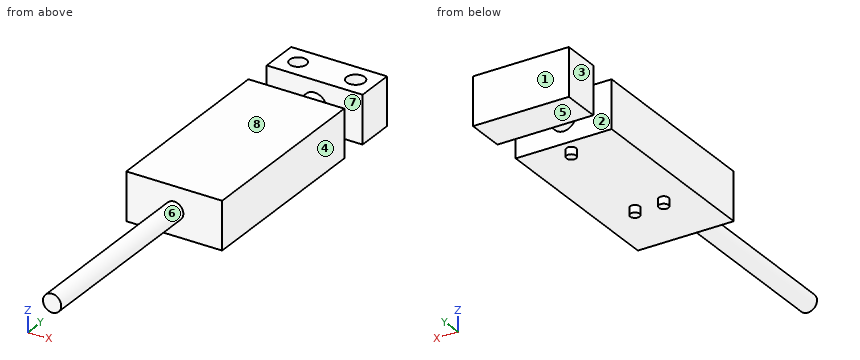
```python
from build123d import *

# Parameters (mm, degrees)
SKETCH1_W           = 200
SKETCH1_H           = 400
BOSS_EXTRUDE1_DEPTH = 100
SKETCH2_R           = 25
BOSS_EXTRUDE2_DEPTH = 60
SKETCH3_W           = 200
SKETCH3_H           = 100
BOSS_EXTRUDE3_DEPTH = 80
SKETCH4_R           = 17.5
SKETCH4_R_2         = 18.82666719
CUT_EXTRUDE1_DEPTH  = 40
SKETCH5_R           = 19
BOSS_EXTRUDE4_DEPTH = 400
SKETCH7_R           = 10
BOSS_EXTRUDE5_DEPTH = 15


with BuildPart() as part:
    # Sketch1 → Boss-Extrude1 (new body)
    with BuildSketch(Plane.XY):
        Rectangle(SKETCH1_W, SKETCH1_H)
    extrude(amount=BOSS_EXTRUDE1_DEPTH)

    # Sketch2 → Boss-Extrude2 (add)
    with BuildSketch(Plane(origin=(0, 200, 0), x_dir=(1, 0, 0), z_dir=(0, 1, 0))):
        with Locations(Location((0, -50, 0), (0, 0, 90))):
            Circle(SKETCH2_R)
    extrude(amount=BOSS_EXTRUDE2_DEPTH)

    # Sketch3 → Boss-Extrude3 (add)
    with BuildSketch(Plane(origin=(0, 260, 0), x_dir=(1, 0, 0), z_dir=(0, 1, 0))):
        with Locations((0, -50)):
            Rectangle(SKETCH3_W, SKETCH3_H)
    extrude(amount=BOSS_EXTRUDE3_DEPTH)

    # Sketch4 → Cut-Extrude1 (cut)
    with BuildSketch(Plane.XY.offset(100)):
        with Locations((-60, 300)):
            Circle(SKETCH4_R)
        with Locations((60, 300)):
            Circle(SKETCH4_R_2)
    extrude(amount=-CUT_EXTRUDE1_DEPTH, mode=Mode.SUBTRACT)

    # Sketch5 → Boss-Extrude4 (add)
    with BuildSketch(Plane.XZ.offset(200)):
        with Locations(Location((0, 50, 0), (0, 0, 270))):
            Circle(SKETCH5_R)
    extrude(amount=BOSS_EXTRUDE4_DEPTH)

    # Sketch7 → Boss-Extrude5 (add)
    with BuildSketch(Plane(origin=(0, 0, 0), x_dir=(-1, 0, 0), z_dir=(0, 0, -1))):
        with Locations(Location((0, 175, 0), (0, 0, 180))):
            Circle(SKETCH7_R)
        with Locations(Location((-20, -65, 0), (0, 0, 180))):
            Circle(SKETCH7_R)
        with Locations(Location((40, -65, 0), (0, 0, 180))):
            Circle(SKETCH7_R)
    extrude(amount=BOSS_EXTRUDE5_DEPTH)


solid = part.part
```
Could you check a few things on this model? Use its own coordinates, in mm. Face numbers are marked on the shaded views. A direction names the side the tool comes from. Coordinates: 2 decimals unless noted, no trailing zeros. Write each loop counter-clockwise with the first axis right and the second up, starting at its lowest first coordinate (ties: lowest second). Pieces come first, ordered by that corner, then holes. Notation, with made-up numbers: (88.25, -13) - (98.25, -13) arc R33 cw to (98.25, 25) - close; hole circle Ø7 at (4.5, 39.5). An arc over 180 degrees is marked (long way). Use a Markdown table: item, result.
Q1. Imagine slicing it at B-B (x = 0). List the corners of the cut face in (y, z) for me.
Geometry check:
| item | result |
|---|---|
| outline | (-600, 31) - (-200, 31) - (-200, 0) - (165, 0) - (165, -15) - (185, -15) - (185, 0) - (200, 0) - (200, 25) - (260, 25) - (260, 0) - (340, 0) - (340, 100) - (260, 100) - (260, 75) - (200, 75) - (200, 100) - (-200, 100) - (-200, 69) - (-600, 69) - close |
Q2. I'm going to push flat-ended pins straight in: pin 1 Ø24 at (x, y) = (27, 292) entering from -Z; pin 2 Ø4 at (x, y) = (-10.5, 218) entering from -Z; pin 3 Ø11.5 at (x, y) = (58, 292) entering from +Z. Where does each tip first touch, or does it pass through?
Geometry check:
| item | result |
|---|---|
| pin 1 | stops at z = 0 |
| pin 2 | stops at z = 26.49 |
| pin 3 | stops at z = 60 |
Q3. Thinking about a two-plate mould opening in Y: for the marked faces 1, 2 and 3, which applies, +Y half, -Y half, draft (parallel to the pull), parting line (faces both ways), or undercut?
Geometry check:
| item | result |
|---|---|
| face 1 | +Y half |
| face 2 | undercut |
| face 3 | draft |
Q4. Imagine slicing it at C-C (y = 175). List the corners of the cut face in (x, z) for me, and give its area (3 significant figures).
Geometry check:
| item | result |
|---|---|
| outline | (-100, 0) - (-10, 0) - (-10, -15) - (10, -15) - (10, 0) - (100, 0) - (100, 100) - (-100, 100) - close |
| area | 20,300 mm2 |
Q5. Imagine slicing it at A-A (x = -60). List the corners of the cut face in (y, z) for me.
Geometry check:
| item | result |
|---|---|
| outline | (-200, 0) - (200, 0) - (200, 100) - (-200, 100) - close; (260, 0) - (340, 0) - (340, 100) - (317.5, 100) - (317.5, 60) - (282.5, 60) - (282.5, 100) - (260, 100) - close |
Q6. Which directions (+Z, -Z, +X, -X, +Y, -Y) give clear straight access to the entire face, cutting with the end or side of a thin tool? Please do the marked faces 4, 5, 6, 7 and 8.
Geometry check:
| item | result |
|---|---|
| face 4 | +Z, -Z, +X, +Y, -Y |
| face 5 | -Z, +X, -X, +Y |
| face 6 | -Y |
| face 7 | none |
| face 8 | +Z, +X, -X, +Y, -Y |
Q7. Please list where these lines run through material, in increasing order: L1, parallel to Y at x = 60, z = 78; L2, parallel to Y at x = -60, z = 71.5; L3, parallel to Y at x = 24, z = 13.5.
Geometry check:
| item | result |
|---|---|
| L1 | y = -200 to 200, 260 to 281.17, 318.83 to 340 |
| L2 | y = -200 to 200, 260 to 282.5, 317.5 to 340 |
| L3 | y = -200 to 200, 260 to 340 |
Q8. Imagine slicing it at D-D (x = 60). List the corners of the cut face in (y, z) for me, and give its area (3 significant figures).
Geometry check:
| item | result |
|---|---|
| outline | (-200, 0) - (200, 0) - (200, 100) - (-200, 100) - close; (260, 0) - (340, 0) - (340, 100) - (318.83, 100) - (318.83, 60) - (281.17, 60) - (281.17, 100) - (260, 100) - close |
| area | 46,500 mm2 |
